Input: part model. Units: mm. Frame: model coordinates. A direction names the side the tool comes from. Give positions to 0.01 mm unless a question says otherwise; leave off trailing zeros. Loops run counter-clockwise (first coordinate to the right, second up) from the corner with the lowest first, then second, coordinate; pieces in that order, holes last. Notation, with made-up numbers: (35, 23) -> (53, 23) arc R25 cw to (53, 61) -> close; hole circle Ø7 at (37.25, -16.75). An arc over 180 degrees is marked (long way). Answer as a JSON object with one key per item and string values. Group by question number.
```python
from build123d import *
from build123d import SkipClean  # not in build123d's __all__

# Parameters (mm, degrees)
F0_R     = 7.25
F1_DEPTH = 8.5
F2_R     = 5.75
F3_DEPTH = 4.25
F5_DEPTH = 25


with BuildPart() as f1:
    # F0 (on Top) → F1 (new body)
    with BuildSketch(Plane.XY):
        Circle(F0_R)
    extrude(amount=F1_DEPTH)

    # F2 (on face) → F3 (cut)
    with BuildSketch(Plane.XY.offset(8.5)):
        Circle(F2_R)
    extrude(amount=-F3_DEPTH, mode=Mode.SUBTRACT)

    # F4 (on Right) → F5 (cut)
    with BuildSketch(Plane.YZ):
        with BuildLine():
            Line((-3, 9.0031314455), (-3, 7.25))
            ThreePointArc((-3, 7.25), (0, 4.25), (3, 7.25))
            Line((3, 7.25), (3, 9.0439899638))
            Line((3, 9.0439899638), (-3, 9.0031314455))
        make_face()
    with SkipClean():  # cleaning this boolean's faces spoils the solid; the shape is the same uncleaned
        extrude(amount=-F5_DEPTH, mode=Mode.SUBTRACT)


solid = f1.part
```
Q1. Ray query, probe 1 along Z at (x, y) = (-0.5, -3); probe 2 along Y at (x, z) = (5, 7.75); probe 3 along Y at (x, z) = (-0.75, 6). Return the intervals inside material, ascending.
Q2. Section B-B on y = -3.75. Return the cut outline in (x, z).
Q3. Section C-C on z = 5. Return the cut outline in (x, y).
Q4. Set-up query: faces 1 (the face through (0, 0, 4.25)), 2 (the face through (6.697, -2.777, 4.19)), 3 (the face through (-6, 3, 8)). Return all of +Z, -Z, +X, -X, +Y, -Y with unobstructed straight access to the full face (end or side cutting, diameter ignored); none if empty.
Q5. Pin query (flat end, axial travel): pin 1 Ø1.5 at (x, z) = (2, 5.5) entering from -Y; pin 2 Ø3 at (x, z) = (-2, 5) entering from -Y; pin 3 Ø4 at (x, y) = (-2.5, 1) entering from +Z. Return the tip coordinate at first contact, or that it passes through.
Q6. Section A-A on x = 0. Return the cut outline in (y, z), then the cut area to 3 significant figures.
Numbers:
{
 "1": {"probe 1": "z = 0 to 4.25", "probe 2": "y = -5.25 to -2.84, 2.84 to 5.25", "probe 3": "y = -7.21 to -5.7, 5.7 to 7.21"},
 "2": {"outline": "(-6.2, 0) -> (6.2, 0) -> (6.2, 8.5) -> (4.36, 8.5) -> (4.36, 4.25) -> (-4.36, 4.25) -> (-4.36, 8.5) -> (-6.2, 8.5) -> close"},
 "3": {"outline": "(-6.97, -1.98) arc R7.25 ccw (long way) to (-6.97, 1.98) -> (-5.4, 1.98) arc R5.75 cw (long way) to (-5.4, -1.98) -> close"},
 "4": {"face 1": "+Z", "face 2": "+Z, -Z", "face 3": "+Z, -X"},
 "5": {"pin 1": "stops at y = -7.14", "pin 2": "stops at y = -7.23", "pin 3": "stops at z = 4.25"},
 "6": {"outline": "(-7.25, 0) -> (7.25, 0) -> (7.25, 8.5) -> (5.75, 8.5) -> (5.75, 4.25) -> (-5.75, 4.25) -> (-5.75, 8.5) -> (-7.25, 8.5) -> close", "area": "74.4 mm²"}
}
